Model file for the job. Use its own axes, mm. A direction names the side the tool comes from. Coordinates: 2 decimals unless noted, no trailing zeros. Write each loop counter-clockwise with the first axis right and the second up, starting at its lowest first coordinate (ties: lowest second). Pieces come first, ordered by that corner, then holes. Notation, with made-up numbers: M 9.5,29 L 57.5,29 A33 ccw 57.5,63 Z; hole C 7,74 d6. An arc over 180 degrees is marked long. Put each result on its own line as item: value. Start each with the question number.
Q1. Which spindle directions (+Z, -Z, +X, -X, +Y, -Y) get a long thin tool onto all of the face, cutting with end or side? Do faces 4 (the flat face through (-2, 0, 2.5)), 5 (the flat face through (-64, 7, 0)). Say none if no direction does.
Q2. Cut at B-B (x = 69). Write the cut outline in (y, z).
Q3. Drill centre lines: line 1 along X through (y, z) = (-0.5, 1.45); line 2 along Y through (x, z) = (80, 1.75); line 3 along X through (y, z) = (-3, 2.2). Where is each one in solid material? Low to high.
Q4. Cut at C-C (z = 0.3). Write the cut outline in (x, y).
Q5. Pull direction Y, two halves, no side cores. Call faces 1 (the cylindrical face through (-90, 0, 0)), 2 (the flat face through (-2, -20, 0)), 3 (the flat face through (-2, 0, -2.5)): pulls with the +Y half, pulls with the -Y half, needs draft (parallel to the pull), parting line crosses it, or undercut.
Q6. Cut at D-D (x = 42). Write the cut outline in (y, z), then the cut area to 3 significant figures.
Q7. Cut at A-A (y = 0). Write the cut outline in (x, z), then the cut area to 3 significant figures.
```python
from build123d import *

# Parameters (mm, degrees)
PLAT_W                       = 40
PLAT_H                       = 5
EL_MENT_M_CANO_SOUD_1_DEPTH  = 230
ENL_V_MAT_EXTRU_1_DEPTH      = 3.5
ENL_V_MAT_EXTRU_1_DEPTH_BACK = 3.5


with BuildPart() as part:
    # plat → Elément mécano-soudé1 (new body)
    with BuildSketch(Plane.YZ.offset(-115)):
        Rectangle(PLAT_W, PLAT_H)
    extrude(amount=EL_MENT_M_CANO_SOUD_1_DEPTH)

    # Esquisse2 → Enlèv. mat.-Extru.1 (cut, two sides)
    with BuildSketch(Plane.XY) as enl_v_mat_extru_1_sk:
        with BuildLine():
            Line((-83, 7), (-45, 7))
            ThreePointArc((-45, 7), (-38, 0), (-45, -7))
            Line((-45, -7), (-83, -7))
            ThreePointArc((-83, -7), (-90, 0), (-83, 7))
        make_face()
        with BuildLine():
            Line((83, 7), (45, 7))
            ThreePointArc((45, 7), (38, 0), (45, -7))
            Line((45, -7), (83, -7))
            ThreePointArc((83, -7), (90, 0), (83, 7))
        make_face()
    extrude(amount=ENL_V_MAT_EXTRU_1_DEPTH, mode=Mode.SUBTRACT)
    extrude(enl_v_mat_extru_1_sk.sketch, amount=-ENL_V_MAT_EXTRU_1_DEPTH_BACK, mode=Mode.SUBTRACT)


solid = part.part
```
Computed values:
1. face 4: +Z, +X, -X, +Y, -Y
1. face 5: +Z, -Z
2. outline: M -20,-2.5 L -7,-2.5 L -7,2.5 L -20,2.5 Z; M 7,-2.5 L 20,-2.5 L 20,2.5 L 7,2.5 Z
3. line 1: -115 to -89.98, -38.02 to 38.02, 89.98 to 115
3. line 2: -20 to -7, 7 to 20
3. line 3: -115 to -89.32, -38.68 to 38.68, 89.32 to 115
4. outline: M -115,-20 L 115,-20 L 115,20 L -115,20 Z; hole M -83,-7 L -45,-7 A7 ccw -45,7 L -83,7 A7 ccw Z; hole M 45,-7 L 83,-7 A7 ccw 83,7 L 45,7 A7 ccw Z
5. face 1: undercut
5. face 2: pulls with the -Y half
5. face 3: needs draft
6. outline: M -20,-2.5 L -6.32,-2.5 L -6.32,2.5 L -20,2.5 Z; M 6.32,-2.5 L 20,-2.5 L 20,2.5 L 6.32,2.5 Z
6. area: 137 mm2
7. outline: M -115,-2.5 L -90,-2.5 L -90,2.5 L -115,2.5 Z; M -38,-2.5 L 38,-2.5 L 38,2.5 L -38,2.5 Z; M 90,-2.5 L 115,-2.5 L 115,2.5 L 90,2.5 Z
7. area: 630 mm2
